```python
from build123d import *

# Parameters (mm, degrees)
SKETCH1_R           = 6.35
BOSS_EXTRUDE1_DEPTH = 12.7


with BuildPart() as part:
    # Sketch1 → Boss-Extrude1 (new body)
    with BuildSketch(Plane.XY):
        with BuildLine():
            Line((129.803523023, 13.72866743), (129.803523023, 32.77866743))
            Line((129.803523023, 32.77866743), (104.403523023, 32.77866743))
            Line((104.403523023, 32.77866743), (89.290523023, 32.77866743))
            Line((89.290523023, 32.77866743), (51.190523023, 32.77866743))
            Line((51.190523023, 32.77866743), (44.078523023, 32.77866743))
            Line((44.078523023, 32.77866743), (42.173523023, 32.77866743))
            ThreePointArc((42.173523023, 32.77866743), (0.864344867, 49.889489273), (-16.246476977, 91.19866743))
            Line((-16.246476977, 91.19866743), (-16.246476977, 115.32866743))
            Line((-16.246476977, 115.32866743), (-18.528129693, 124.368857105))
            ThreePointArc((-18.528129693, 124.368857105), (-35.296476977, 134.37866743), (-52.064824261, 124.368857105))
            Line((-52.064824261, 124.368857105), (-54.346476977, 115.32866743))
            Line((-54.346476977, 115.32866743), (-54.346476977, 91.438289009))
            ThreePointArc((-54.346476977, 91.438289009), (-63.850433524, 50.845698757), (-90.386686587, 18.691214671))
            Line((-90.386686587, 18.691214671), (-171.948476977, -43.42133257))
            Line((-171.948476977, -43.42133257), (-87.747476977, -43.42133257))
            Line((-87.747476977, -43.42133257), (-87.747476977, -49.77133257))
            Line((-87.747476977, -49.77133257), (-61.229320991, -49.77133257))
            Line((-61.229320991, -49.77133257), (-16.694588765, -49.77133257))
            Line((-16.694588765, -49.77133257), (64.652523023, -49.77133257))
            Line((64.652523023, -49.77133257), (64.652523023, -43.42133257))
            Line((64.652523023, -43.42133257), (129.803523023, -43.42133257))
            Line((129.803523023, -43.42133257), (129.803523023, -24.37133257))
            Line((129.803523023, -24.37133257), (139.328523023, -24.37133257))
            Line((139.328523023, -24.37133257), (139.328523023, 13.72866743))
            Line((139.328523023, 13.72866743), (129.803523023, 13.72866743))
        make_face()
        with Locations((-35.296476977, 115.32866743)):
            Circle(SKETCH1_R, mode=Mode.SUBTRACT)
    extrude(amount=BOSS_EXTRUDE1_DEPTH)


solid = part.part
```
Check sheet for the modelled part. Datum: model origin and axes. Units: mm. A direction names the side the tool comes from. Give positions to 0.01 mm unless a question says otherwise; leave off trailing zeros. Write each loop counter-clockwise with the first axis right and the second up, starting at its lowest first coordinate (ties: lowest second). Pieces come first, ordered by that corner, then holes. Notation, with made-up numbers: (76, 65) -> (86, 65) arc R21 ccw to (86, 89) -> close; hole circle Ø7 at (-5, 16.25). An arc over 180 degrees is marked (long way). Use CSV: the item, a comma, the result in double quotes. Start each with the question number.
Q1. Scan lines: line 1 along Y through (x, z) = (41, 12); line 2 along Y through (x, z) = (67, 11.5); line 3 along X through (y, z) = (-8.5, 1). Record each from-to range of solid material in increasing order.
Q2. Cross-section at B-B on x = 113. Enter the section's corners in (y, z), and give its area (3 significant figures).
Q3. Depth check by flat-ended pin: P1, Ø5, axis at y = -48, z = 6.5, coming from the -X side; P2, Ø4, axis at x = 95.5, z = 4, coming from the -Y side; P3, Ø4, axis at y = 64.5, z = 8.5, coming from the +X side; P4, Ø1, axis at x = -113, y = 4, coming from the +Z side. Enter the tip coordinate at first touch or a pass-through.
Q4. Tool access check on faces 1 (the flat face through (139.329, -6, 6)), 2 (the flat face through (97, -43.421, 6)), 3 (the cylindrical face through (-36.67, 109.13, 6.26)), 4 (the flat face through (-54.346, 104, 6)), 5 (the flat face through (87, 32.779, 6)). Record the directions out of +Z, -Z, +X, -X, +Y, -Y that give a thin tool (end or side, any length) a straight path to the whole face; none if there is none.
Q5. Cross-section at A-A on z = 9.75. Enter the section's corners in (x, y), and give its area (3 significant figures).
Q6. Cross-section at C-C on y = 83. Enter the section's corners in (x, z).
Working result:
1,line 1,"y = -49.77 to 32.79"
1,line 2,"y = -43.42 to 32.78"
1,line 3,"x = -126.09 to 139.33"
2,outline,"(-43.42, 0) -> (32.78, 0) -> (32.78, 12.7) -> (-43.42, 12.7) -> close"
2,area,"968 mm^2"
3,P1,"stops at x = -87.75"
3,P2,"stops at y = -43.42"
3,P3,"stops at x = -8.71"
3,P4,"passes through"
4,face 1,"+Z, -Z, +X, +Y, -Y"
4,face 2,"+Z, -Z, +X, -Y"
4,face 3,"+Z, -Z"
4,face 4,"+Z, -Z, -X, +Y"
4,face 5,"+Z, -Z, +X, +Y"
5,outline,"(-171.95, -43.42) -> (-87.75, -43.42) -> (-87.75, -49.77) -> (64.65, -49.77) -> (64.65, -43.42) -> (129.8, -43.42) -> (129.8, -24.37) -> (139.33, -24.37) -> (139.33, 13.73) -> (129.8, 13.73) -> (129.8, 32.78) -> (42.17, 32.78) arc R58.42 cw to (-16.25, 91.2) -> (-16.25, 115.33) -> (-18.53, 124.37) arc R19.05 ccw to (-52.06, 124.37) -> (-54.35, 115.33) -> (-54.35, 91.44) arc R91.44 cw to (-90.39, 18.69) -> close; hole circle Ø12.7 at (-35.3, 115.33)"
5,area,"25,200 mm^2"
6,outline,"(-54.74, 0) -> (-15.67, 0) -> (-15.67, 12.7) -> (-54.74, 12.7) -> close"
